Autodesk Inventor part; units mm, degrees
ref_plane "YZ Plane" through (0, 0, 0) normal (1, 0, 0) x (0, 1, 0)
ref_plane "XZ Plane" through (0, 0, 0) normal (0, 1, 0) x (-1, 0, 0)
ref_plane "XY Plane" through (0, 0, 0) normal (0, 0, 1) x (1, 0, 0)
sketch "Sketch1" plane through (0, 0, 0) normal (0, 1, 0) x (-1, 0, 0)
  line L0 (2.2361, -2) -> (-2.2361, -2)
  line L1 (2.2361, 2) -> (-2.2361, 2)
  arc A0 (2.2361, -2) -> (2.2361, 2) centre (0, 0) ccw
  arc A1 (-2.2361, 2) -> (-2.2361, -2) centre (0, 0) ccw
  circle A2 centre (0, 0) radius 5
  dimension "d1" = 2
  dimension "d2" = 2
  dimension "d3" = 10
  dimension "d20" = 3
  dimension "d21" = 3
extrude "Extrusion1" add sketch "Sketch1" along normal blind 5
sketch "Sketch2" plane through (0, 0, 0) normal (0, -1, 0) x (1, 0, 0)
  circle A0 centre (0, 0) radius 5
  dimension "d19" = 10
extrude "Extrusion2" add sketch "Sketch2" along normal blind 5
sketch "Sketch3" plane through (0, -5, 0) normal (0, -1, 0) x (1, 0, 0)
  circle A0 centre (0, 0) radius 2.625
  line L0 (1.2228, 2.3228) -> (1.2228, 1.2228)
  line L1 (1.2228, -1.2228) -> (1.2228, -2.3228)
  line L2 (2.3228, -1.2228) -> (1.2228, -1.2228)
  line L3 (-1.2228, -1.2228) -> (-2.3228, -1.2228)
  line L4 (2.3228, 1.2228) -> (1.2228, 1.2228)
  line L5 (-1.2228, 1.2228) -> (-2.3228, 1.2228)
  line L6 (-1.2228, 2.3228) -> (-1.2228, 1.2228)
  line L7 (-1.2228, -1.2228) -> (-1.2228, -2.3228)
  dimension "d10" = 5.25
  dimension "d22" = 1.1
  dimension "d23" = 1.1
  dimension "d24" = 1.1
  dimension "d25" = 1.1
  dimension "d26" = 1.1
  dimension "d27" = 1.1
  dimension "d28" = 1.1
  dimension "d29" = 1.1
extrude "Extrusion3" cut sketch "Sketch3" against normal blind 5 contours A0 L2 L1 L7 L3 L5 L6 L0 L4
fillet "Fillet2" radius 0.5 12 edges at (2.625, -5, 0) (1.7728, -5, 1.2228) (1.2228, -5, 1.7728) (0, -5, 2.625) (-1.2228, -5, 1.7728) (-2.625, -5, 0) (-1.7728, -5, 1.2228) (-1.7728, -5, -1.2228) (-1.2228, -5, -1.7728) (0, -5, -2.625) (1.7728, -5, -1.2228) (1.2228, -5, -1.7728)
equation "\"d23\" = d22"
equation "\"d24\" = d22"
equation "\"d25\" = d22"
equation "\"d26\" = d22"
equation "\"d27\" = d22"
equation "\"d28\" = d22"
equation "\"d29\" = d22"
properties part number "dif-coupler"
Input: part model. Units: mm. Frame: model coordinates. A direction names the side the tool comes from. Give positions to 0.01 mm unless a question says otherwise; leave off trailing zeros. Order: outer loops, then holes, each group sorted by start corner. A loop starts at its lowest first (then second) coordinate and runs counter-clockwise, first axis right, second up. Notation, with made-up numbers: M 12,4 L 30,4 A26 ccw 30,20 Z; hole C 74.25,46.25 d3. An arc over 180 degrees is marked long. Answer as a JSON object with one key per item and string values.
1. Ray query, line 1 (X direction, y = -2.75, z = 0) (3 decimals); line 2 (X direction, y = -3.25, z = 4); line 3 (X direction, y = 1.5, z = -0.25). Return the intervals inside material, ascending. Write a range as [from, to].
Result sheet:
{"line 1": "[-5, -2.625], [2.625, 5]", "line 2": "[-3, 3]", "line 3": "[-4.99, -2.99], [2.99, 4.99]"}
2. First-contact query: P1, Ø1, axis at y = 4, z = -1.5, coming from the +X side; P2, Ø1.4, axis at x = -2, z = 0.5, coming from the +Y side; P3, Ø0.5, axis at x = -2, y = -3, coming from the -Z side. Flat tips, straight axial feed; report the tip coordinate or a pass-through.
Result sheet:
{"P1": "x = 4.9", "P2": "y = 0", "P3": "z = -4.68"}
3. Pull-direction query (Z, two-part tool) for faces 5 (the flat face through (2, -5, -2)), 6 (the flat face through (0, 2, 2)); classes: +Z half, -Z half, draft (parallel to the pull), parting line (faces both ways), or undercut.
Result sheet:
{"face 5": "draft", "face 6": "undercut"}
4. Reachability of faces 1 (the cylindrical face through (-0.018, -2.282, -2.625)), 2 (the flat face through (0.1, 5, -2.2)), 3 (the flat face through (-2, -2, 1.223)), 4 (the cylindrical face through (-3, 2, 0)) from +Z, -Z, +X, -X, +Y, -Y: full face, straight path, thin tool, end or side. Return the list, or none.
Result sheet:
{"face 1": "-Y", "face 2": "+Z, -Z, +X, -X, +Y", "face 3": "+Y, -Y", "face 4": "+Y"}
5. Cut plane A-A, the plane x = 0. Output: boundary loops of the cut face in (y, z) (3 decimals).
Result sheet:
{"outline": "M -5,-5 L 5,-5 L 5,-2 L 0,-2 L 0,-2.625 L -4.5,-2.625 A0.5 ccw -5,-3.125 Z; M -5,3.125 A0.5 ccw -4.5,2.625 L 0,2.625 L 0,2 L 5,2 L 5,5 L -5,5 Z"}
6. Cut plane C-C, the plane y = -2.75. Output: boundary loops of the cut face in (x, z) (3 decimals), and give its area (3 significant figures).
Result sheet:
{"outline": "C 0,0 d10; hole M -2.323,-1.223 L -1.223,-1.223 L -1.223,-2.323 A2.625 ccw 1.223,-2.323 L 1.223,-1.223 L 2.323,-1.223 A2.625 ccw 2.323,1.223 L 1.223,1.223 L 1.223,2.323 A2.625 ccw -1.223,2.323 L -1.223,1.223 L -2.323,1.223 A2.625 ccw Z", "area": "59.8 mm²"}
7. Cut plane B-B, the plane z = 0. Output: boundary loops of the cut face in (x, y) (3 decimals), and give its area (3 significant figures).
Result sheet:
{"outline": "M -5,-5 L -3.125,-5 A0.5 ccw -2.625,-4.5 L -2.625,0 L -3,0 L -3,5 L -5,5 Z; M 2.625,-4.5 A0.5 ccw 3.125,-5 L 5,-5 L 5,5 L 3,5 L 3,0 L 2.625,0 Z", "area": "43.6 mm²"}
8. Cut plane D-D, the plane y = 0.25. Output: boundary loops of the cut face in (x, z).
Result sheet:
{"outline": "C 0,0 d10; hole M -2.24,-2 L 2.24,-2 A3 ccw 2.24,2 L -2.24,2 A3 ccw Z"}
